Here's how the part is built. I have some questions about the finished solid (model axes, mm). A direction names the side the tool comes from. Round coordinates to 2 decimals unless told otherwise and drop trailing zeros. Order: outer loops, then holes, each group sorted by start corner. A loop starts at its lowest first (then second) coordinate and runs counter-clockwise, first axis right, second up. Notation, with made-up numbers: (16.25, 81.5) -> (24.25, 81.5) arc R18 cw to (24.25, 88.5) -> close; hole circle Ø3 at (61.25, -12.5). An arc over 180 degrees is marked (long way). Use a Markdown table: item, result. Add a question column.
(1) I want a section at B-B, the plane z = 2.25. Please give me the cut outline in (x, y).
(2) I'm going to push flat-ended pins straight in: P1, Ø1, axis at y = -1, z = -6, coming from the -X side; P2, Ø11.5, axis at x = -4, z = 0, coming from the -Y side; P3, Ø2.5, axis at x = 0, y = -1.5, coming from the +Z side. Where does each tip first touch, or does it pass through?
(3) I want a section at C-C, the plane y = -1. Please give me the cut outline in (x, z).
(4) I want a section at A-A, the plane x = -12.5. Please give me the cut outline in (y, z), then the cut area to 3 significant figures.
(5) If I drill on probe 1 along Y at (x, z) = (19, -10.25); probe 2 along Z at (x, y) = (8, -0.25), over which ranges is the centre line in solid material (lowest first)?
(6) On a 3-axis mill with a long thin cutter (end or side, diameter ignored), from which of +Z, -Z, +X, -X, +Y, -Y can I reach the whole of each face in a straight line? I mean faces 1 (the face through (35, 1, 0)), 2 (the face through (0, -1, -10.5)). Say none if no direction works.
Autodesk Inventor part; units mm, degrees
ref_plane "YZ Plane" through (0, 0, 0) normal (1, 0, 0) x (0, 1, 0)
ref_plane "XZ Plane" through (0, 0, 0) normal (0, 1, 0) x (-1, 0, 0)
ref_plane "XY Plane" through (0, 0, 0) normal (0, 0, 1) x (1, 0, 0)
sketch "Sketch1" plane through (0, 0, 0) normal (0, 1, 0) x (-1, 0, 0)
  line L0 (35, 12.5) -> (-35, 12.5)
  line L1 (-35, 12.5) -> (-35, -12.5)
  line L2 (-35, -12.5) -> (35, -12.5)
  line L3 (35, -12.5) -> (35, 12.5)
  line L4 (35, 12.5) -> (-35, -12.5) construction
  line L5 (-35, 12.5) -> (35, -12.5) construction
  point P0 (0, 0)
  dimension "d0" = 70
  dimension "d1" = 25
extrude "Extrusion1" add sketch "Sketch1" along normal blind 2
sketch "Sketch2" plane through (0, 0, 0) normal (0, -1, 0) x (1, 0, 0)
  line L0 (35, 12.5) -> (35, -12.5)
  line L1 (35, -12.5) -> (-35, -12.5)
  line L2 (-35, -12.5) -> (35, -12.5)
  line L3 (35, -12.5) -> (35, -10.5)
  line L4 (35, -10.5) -> (-35, -10.5)
  line L5 (-35, -10.5) -> (-35, -12.5)
  point P0 (0, 0)
  dimension "d7" = 2
extrude "Extrusion2" add sketch "Sketch2" along normal blind 3
properties part number "SP46V1 Felpa Roldana" material "Fabric"
Taken from the geometry:
| question | item | result |
|---|---|---|
| 1 | outline | (-35, 0) -> (35, 0) -> (35, 2) -> (-35, 2) -> close |
| 2 | P1 | passes through |
| 2 | P2 | stops at y = 0 |
| 2 | P3 | stops at z = -10.5 |
| 3 | outline | (-35, -12.5) -> (35, -12.5) -> (35, -10.5) -> (-35, -10.5) -> close |
| 4 | outline | (-3, -12.5) -> (2, -12.5) -> (2, 12.5) -> (0, 12.5) -> (0, -10.5) -> (-3, -10.5) -> close |
| 4 | area | 56.0 mm2 |
| 5 | probe 1 | y = 0 to 2 |
| 5 | probe 2 | z = -12.5 to -10.5 |
| 6 | face 1 | +Z, -Z, +X, +Y, -Y |
| 6 | face 2 | +Z, +X, -X, -Y |
